Read the model definition and answer for the solid it produces. Units are mm, in the model's axes. A direction names the side the tool comes from. Give positions to 0.01 mm unless a question says otherwise; leave off trailing zeros. Write each loop counter-clockwise with the first axis right and the second up, starting at its lowest first coordinate (ties: lowest second). Pieces come first, ordered by that corner, then holes. Notation, with made-up numbers: (33.5, 84.5) -> (63.5, 84.5) arc R17 cw to (63.5, 100.5) -> close; hole circle Ø10 at (-39.5, 47.25). An arc over 180 degrees is marked (long way). Use a Markdown table: item, result.
from build123d import *

# Parameters (mm, degrees)
SKETCH1_R           = 17.5
BOSS_EXTRUDE1_DEPTH = 15
BOSS_EXTRUDE2_DEPTH = 2
CUT_EXTRUDE1_REACH  = 19
SKETCH3_R           = 3.25
SKETCH4_R           = 1
CUT_EXTRUDE2_DEPTH  = 5
CIRPATTERN1_COUNT   = 4
SKETCH5_R           = 1
CUT_EXTRUDE3_DEPTH  = 2
CIRPATTERN2_COUNT   = 4
SKETCH6_R           = 7.5
CUT_EXTRUDE4_DEPTH  = 5
CUT_EXTRUDE6_START  = -4
SKETCH7_R           = 17.5
SKETCH7_R_2         = 12.5
CUT_EXTRUDE6_DEPTH  = 0.2
FILLET1_R           = 2
CUT_EXTRUDE7_DEPTH  = 3


with BuildPart() as part:
    # Sketch1 → Boss-Extrude1 (new body)
    with BuildSketch(Plane(origin=(0, 0, 0), x_dir=(1, 0, 0), z_dir=(0, 1, 0))):
        Circle(SKETCH1_R)
    extrude(amount=BOSS_EXTRUDE1_DEPTH)

    # Sketch2 → Boss-Extrude2 (add)
    with BuildSketch(Plane(origin=(0, 15, 0), x_dir=(1, 0, 0), z_dir=(0, 1, 0))):
        Polygon((7.3, 0), (3.65, 6.321985448), (-3.65, 6.321985448), (-7.3, 0), (-3.65, -6.321985448), (3.65, -6.321985448), align=None)
    extrude(amount=BOSS_EXTRUDE2_DEPTH)

    # Sketch3 → Cut-Extrude1 (cut, up to next)
    with BuildSketch(Plane.XZ, mode=Mode.PRIVATE) as cut_extrude1_sk1:
        Circle(SKETCH3_R)
    cut_extrude1_tool1 = extrude(cut_extrude1_sk1.sketch, amount=-CUT_EXTRUDE1_REACH, mode=Mode.PRIVATE) & part.part
    add(cut_extrude1_tool1.solids().sort_by_distance((0, 0, 0))[0], mode=Mode.SUBTRACT)

    # Sketch4 → Cut-Extrude2 (cut)
    with BuildSketch(Plane.XZ):
        with Locations((0, 9.5)):
            Circle(SKETCH4_R)
    cut_extrude2 = extrude(amount=-CUT_EXTRUDE2_DEPTH, mode=Mode.SUBTRACT)

    # CirPattern1: Cut-Extrude2 ×4 about axis
    cirpattern1_axis = Axis((0, 0, 0), (0, 1, 0))
    for i in range(1, CIRPATTERN1_COUNT):
        add(cut_extrude2.rotate(cirpattern1_axis, i * 360 / CIRPATTERN1_COUNT), mode=Mode.SUBTRACT)

    # Sketch5 → Cut-Extrude3 (cut)
    with BuildSketch(Plane(origin=(0, 15, 0), x_dir=(1, 0, 0), z_dir=(0, 1, 0))):
        with Locations((0, 14.5)):
            Circle(SKETCH5_R)
    cut_extrude3 = extrude(amount=-CUT_EXTRUDE3_DEPTH, mode=Mode.SUBTRACT)

    # CirPattern2: Cut-Extrude3 ×4 about axis
    cirpattern2_axis = Axis((0, 0, 0), (0, 1, 0))
    for i in range(1, CIRPATTERN2_COUNT):
        add(cut_extrude3.rotate(cirpattern2_axis, i * 360 / CIRPATTERN2_COUNT), mode=Mode.SUBTRACT)

    # Sketch6 → Cut-Extrude4 (cut)
    with BuildSketch(Plane(origin=(0, 15, 0), x_dir=(1, 0, 0), z_dir=(0, 1, 0))):
        Circle(SKETCH6_R)
        Polygon((7.3, 0), (3.65, 6.321985448), (-3.65, 6.321985448), (-7.3, 0), (-3.65, -6.321985448), (3.65, -6.321985448), align=None, mode=Mode.SUBTRACT)
    extrude(amount=-CUT_EXTRUDE4_DEPTH, mode=Mode.SUBTRACT)

    # Sketch7 → Cut-Extrude6 (cut)
    with BuildSketch(Plane(origin=(0, 15, 0), x_dir=(1, 0, 0), z_dir=(0, 1, 0)).offset(CUT_EXTRUDE6_START)):
        Circle(SKETCH7_R)
        Circle(SKETCH7_R_2, mode=Mode.SUBTRACT)
    extrude(amount=-CUT_EXTRUDE6_DEPTH, mode=Mode.SUBTRACT)

    # Fillet1
    fillet1_edges = [part.edges().sort_by_distance(p)[0] for p in [
        (-7.3, 13.5, 0),
        (-3.65, 13.5, 6.321985448),
        (3.65, 13.5, 6.321985448),
        (7.3, 13.5, 0),
        (3.65, 13.5, -6.321985448),
        (-3.65, 13.5, -6.321985448),
    ]]
    fillet(fillet1_edges, radius=FILLET1_R)

    # Sketch8 → Cut-Extrude7 (cut)
    with BuildSketch(Plane(origin=(0, 15, 0), x_dir=(1, 0, 0), z_dir=(0, 1, 0))):
        with BuildLine():
            Line((8.042991645, 14.406952676), (5.21456452, 11.578525551))
            Line((5.21456452, 11.578525551), (11.578525551, 5.21456452))
            Line((11.578525551, 5.21456452), (14.406952676, 8.042991645))
            ThreePointArc((14.406952676, 8.042991645), (11.66726189, 11.66726189), (8.042991645, 14.406952676))
        make_face()
    extrude(amount=-CUT_EXTRUDE7_DEPTH, mode=Mode.SUBTRACT)


solid = part.part
Item 1: A tool of negligible diameter and unlimited length cuts with its end or side. For faces 4 (the face through (10, 5, 0)), 5 (the face through (-13.887, 5.324, 10.648)), 6 (the face through (-0.217, 14.014, -13.524)), 7 (the face through (8, 11, 11)), 8 (the face through (-2, 17, -3)), from which of +Z, -Z, +X, -X, +Y, -Y can it reach the whole face along a straight path? Write none if from no direction.
Return value:
| item | result |
|---|---|
| face 4 | -Y |
| face 5 | +Y, -Y |
| face 6 | +Y |
| face 7 | none |
| face 8 | +Z, -Z, +X, -X, +Y |
Item 2: Each of these flat-tipped pins is pushed along its axis until it touches: P1, Ø1.6, axis at x = 0, z = -14.5, coming from the +Y side; P2, Ø1, axis at y = 7, z = -2.5, coming from the +X side; P3, Ø2, axis at x = 3, y = 12, coming from the +Z side. Where does it stop, or does it pass through?
Return value:
| item | result |
|---|---|
| P1 | y = 13 |
| P2 | x = 17.39 |
| P3 | z = 17.39 |
Item 3: A cutting plane is placed at C-C (z = 4.5). Give the vertices of the cut face in (x, y).
Return value:
| item | result |
|---|---|
| outline | (-16.91, 0) -> (16.91, 0) -> (16.91, 10.8) -> (11.66, 10.8) -> (11.66, 11) -> (16.91, 11) -> (16.91, 15) -> (6, 15) -> (6, 10) -> (4.7, 10) -> (4.7, 17) -> (-4.7, 17) -> (-4.7, 10) -> (-6, 10) -> (-6, 15) -> (-16.91, 15) -> (-16.91, 11) -> (-11.66, 11) -> (-11.66, 10.8) -> (-16.91, 10.8) -> close |
Item 4: Straight lines are drawn through the part: line 1 along Z through (x, y) = (0, 1.45); line 2 along Y through (x, z) = (13.5, -6); line 3 along Z through (x, y) = (3.5, 10.5). For each, find the intervals that lie inside material, in ascending order. Write a range as [from, to].
Return value:
| item | result |
|---|---|
| line 1 | [-17.5, -10.5], [-8.5, -3.25], [3.25, 8.5], [10.5, 17.5] |
| line 2 | [0, 10.8], [11, 15] |
| line 3 | [-17.15, -6.63], [-6.05, 6.05], [6.63, 17.15] |
Item 5: A cutting plane is placed at B-B (y = 1). Give the vertices of the cut face in (x, z), then the cut area to 3 significant figures.
Return value:
| item | result |
|---|---|
| outline | circle Ø35 at (0, 0); hole circle Ø2 at (-9.5, 0); hole circle Ø6.5 at (0, 0); hole circle Ø2 at (0, -9.5); hole circle Ø2 at (0, 9.5); hole circle Ø2 at (9.5, 0) |
| area | 916 mm^2 |
Item 6: For a pull along X with two mould halves and no side action, classify faces 1 (the face through (0, 15, 8)), 2 (the face through (6.649, 13.521, -13.013)), 3 (the face through (-13.887, 12.972, 10.648)) as +X half, -X half, draft (parallel to the pull), parting line (faces both ways), or undercut.
Return value:
| item | result |
|---|---|
| face 1 | draft |
| face 2 | undercut |
| face 3 | parting line |
Item 7: A cutting plane is placed at A-A (y = 11.5). Give the vertices of the cut face in (x, z).
Return value:
| item | result |
|---|---|
| outline | circle Ø35 at (0, 0); (-6.72, -1) -> (-4.23, -5.32) arc R2 ccw to (-2.5, -6.32) -> (2.5, -6.32) arc R2 ccw to (4.23, -5.32) -> (6.72, -1) arc R2 ccw to (6.72, 1) -> (4.23, 5.32) arc R2 ccw to (2.5, 6.32) -> (-2.5, 6.32) arc R2 ccw to (-4.23, 5.32) -> (-6.72, 1) arc R2 ccw to start; hole circle Ø15 at (0, 0); hole circle Ø6.5 at (0, 0) |
Item 8: A cutting plane is placed at D-D (x = -14.5). Give the vertices of the cut face in (y, z), then the cut area to 3 significant figures.
Return value:
| item | result |
|---|---|
| outline | (0, -9.8) -> (10.8, -9.8) -> (10.8, 9.8) -> (0, 9.8) -> close; (11, -9.8) -> (15, -9.8) -> (15, -1) -> (13, -1) -> (13, 1) -> (15, 1) -> (15, 9.8) -> (11, 9.8) -> close |
| area | 286 mm^2 |
